Build history of the part. All positions in model axes, mm. Face numbers are marked on the shaded views. A direction names the side the tool comes from. Give positions to 0.01 mm unless a question says otherwise; leave off trailing zeros. Order: outer loops, then holes, each group sorted by start corner. A loop starts at its lowest first (then second) coordinate and runs counter-clockwise, first axis right, second up. Notation, with made-up numbers: (-17, 17) -> (23, 17) arc R20 cw to (23, 54) -> close; hole circle Ø6 at (-11.75, 15.25). An arc over 180 degrees is marked (long way). Write item = value, one per line. Start each with the question number.
from build123d import *

# Parameters (mm, degrees)
SKETCH1_W           = 140
SKETCH1_H           = 110
BOSS_EXTRUDE1_DEPTH = 5
SKETCH3_W           = 140
SKETCH3_H           = 110
SKETCH3_W_2         = 134
SKETCH3_H_2         = 104
BOSS_EXTRUDE2_DEPTH = 30
CUT_EXTRUDE3_DEPTH  = 5
FILLET1_R           = 3
SKETCH5_R           = 4
CUT_EXTRUDE4_DEPTH  = 2
SKETCH6_R           = 2
CUT_EXTRUDE5_DEPTH  = 5
FILLET2_R           = 10
CUT_EXTRUDE6_DEPTH  = 3
SKETCH9_W           = 32
SKETCH9_H           = 3
CUT_EXTRUDE7_DEPTH  = 3
SKETCH10_W          = 71
SKETCH10_H          = 23
CUT_EXTRUDE8_DEPTH  = 3


with BuildPart() as part:
    # Sketch1 → Boss-Extrude1 (new body)
    with BuildSketch(Plane(origin=(0, 0, 0), x_dir=(1, 0, 0), z_dir=(0, 1, 0))):
        with Locations((70, -55)):
            Rectangle(SKETCH1_W, SKETCH1_H)
    extrude(amount=BOSS_EXTRUDE1_DEPTH)

    # Sketch3 → Boss-Extrude2 (add)
    with BuildSketch(Plane(origin=(0, 5, 0), x_dir=(1, 0, 0), z_dir=(0, 1, 0))):
        with Locations((70, -55)):
            Rectangle(SKETCH3_W, SKETCH3_H)
        with Locations((70, -55)):
            Rectangle(SKETCH3_W_2, SKETCH3_H_2, mode=Mode.SUBTRACT)
    extrude(amount=BOSS_EXTRUDE2_DEPTH)

    # Sketch4 → Cut-Extrude3 (cut)
    with BuildSketch(Plane(origin=(0, 5, 0), x_dir=(1, 0, 0), z_dir=(0, 1, 0))):
        Polygon((23, -6), (23, -23), (6, -23), (6, -87), (23, -87), (23, -104), (117, -104), (117, -87), (134, -87), (134, -23), (117, -23), (117, -6), align=None)
    extrude(amount=-CUT_EXTRUDE3_DEPTH, mode=Mode.SUBTRACT)

    # Fillet1
    fillet1_edges = [part.edges().sort_by_distance(p)[0] for p in [
        (23, 2.5, 6),
        (117, 2.5, 6),
        (134, 2.5, 23),
        (134, 2.5, 87),
        (117, 2.5, 104),
        (23, 2.5, 104),
        (6, 2.5, 87),
        (6, 2.5, 23),
    ]]
    fillet(fillet1_edges, radius=FILLET1_R)

    # Sketch5 → Cut-Extrude4 (cut)
    with BuildSketch(Plane(origin=(0, 5, 0), x_dir=(1, 0, 0), z_dir=(0, 1, 0))):
        with Locations(Location((13, -13, 0), (0, 0, 270))):
            Circle(SKETCH5_R)
        with Locations(Location((13, -97, 0), (0, 0, 270))):
            Circle(SKETCH5_R)
    cut_extrude4 = extrude(amount=-CUT_EXTRUDE4_DEPTH, mode=Mode.SUBTRACT)

    # Sketch6 → Cut-Extrude5 (cut)
    with BuildSketch(Plane(origin=(0, 5, 0), x_dir=(1, 0, 0), z_dir=(0, 1, 0))):
        with Locations(Location((13, -13, 0), (0, 0, 270))):
            Circle(SKETCH6_R)
        with Locations(Location((13, -97, 0), (0, 0, 270))):
            Circle(SKETCH6_R)
    cut_extrude5 = extrude(amount=-CUT_EXTRUDE5_DEPTH, mode=Mode.SUBTRACT)

    # Mirror1: Cut-Extrude4, Cut-Extrude5 across plane
    add(cut_extrude4.mirror(Plane(origin=(70, 0, 0), x_dir=(0, 0, 1), z_dir=(1, 0, 0))), mode=Mode.SUBTRACT)
    add(cut_extrude5.mirror(Plane(origin=(70, 0, 0), x_dir=(0, 0, 1), z_dir=(1, 0, 0))), mode=Mode.SUBTRACT)

    # Fillet2
    fillet2_edges = [part.edges().sort_by_distance(p)[0] for p in [
        (117, 2.5, 23),
        (117, 2.5, 87),
        (23, 2.5, 87),
        (23, 2.5, 23),
    ]]
    fillet(fillet2_edges, radius=FILLET2_R)

    # Sketch8 → Cut-Extrude6 (cut)
    with BuildSketch(Plane(origin=(0, 0, 0), x_dir=(-1, 0, 0), z_dir=(0, 0, -1))):
        Polygon((-127, 31), (-127, 10), (-28, 10), (-28, 28), (-93, 28), (-93, 31), align=None)
    extrude(amount=-CUT_EXTRUDE6_DEPTH, mode=Mode.SUBTRACT)

    # Sketch9 → Cut-Extrude7 (cut)
    with BuildSketch(Plane(origin=(0, 0, 0), x_dir=(-1, 0, 0), z_dir=(0, 0, -1))):
        with Locations((-59, 33.5)):
            Rectangle(SKETCH9_W, SKETCH9_H)
    extrude(amount=-CUT_EXTRUDE7_DEPTH, mode=Mode.SUBTRACT)

    # Sketch10 → Cut-Extrude8 (cut)
    with BuildSketch(Plane.ZY):
        with Locations((55.5, 16.5)):
            Rectangle(SKETCH10_W, SKETCH10_H)
    extrude(amount=-CUT_EXTRUDE8_DEPTH, mode=Mode.SUBTRACT)


solid = part.part
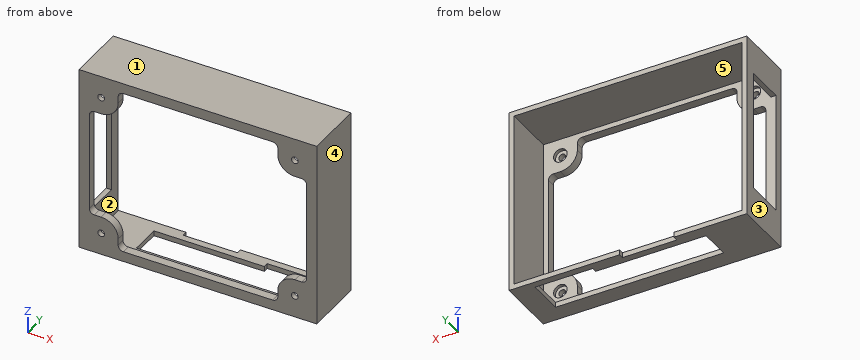
(1) Cut at A-A, the plane z = 35.5. Give the cut face in (x, y).
(2) Mould opens along Z. For the marked faces 1, 2 and 3 say: released by +Z, released by -Z, zero draft, split by the parting line, or undercut.
(3) 3-axis set-ups, long thin cutter, end or side, ignore diameter. For the marked faces 4 and 5: which of +Z, -Z, +X, -X, +Y, -Y reach the whole face in a straight line?
(4) Flat gauge pins, fed straight in: P1, Ø4, axis at y = 28.5, z = 87, coming from the -X side; P2, Ø9, axis at x = 127, z = 97, coming from the +Y side; P3, Ø3, axis at y = 17, z = 81.5, coming from the -X side; P4, Ø2.5, axis at x = 13, z = 97, coming from the -Y side. Where does each tip first touch, or does it go through?
(5) Cut at D-D, the plane x = 30. Give the cut face in (y, z).
(6) Wall check: line 1 (X direction, y = 3.75, z = 97); line 2 (X direction, y = 30, z = 68); line 3 (Z direction, x = 131.5, y = 7). Give the ranges that are in metal, low to high. Write a range as [from, to].
(7) Cut at C-C, the plane x = 49.5. Give the cut face in (y, z).
(8) Cut at B-B, the plane y = 18. Give the cut face in (x, z), plus the area to 3 significant figures.
Results:
q1.outline = (0, 0) -> (6, 0) -> (6, 5) -> (0, 5) -> close; (0, 28) -> (3, 28) -> (3, 35) -> (0, 35) -> close; (134, 0) -> (140, 0) -> (140, 35) -> (137, 35) -> (137, 5) -> (134, 5) -> close
q2.face_1 = released by +Z
q2.face_2 = undercut
q2.face_3 = zero draft
q3.face_4 = +Z, -Z, +X, +Y, -Y
q3.face_5 = +Y
q4.P1 = 0
q4.P2 = 5
q4.P3 = 137
q4.P4 = through
q5.outline = (0, 0) -> (10, 0) -> (10, 3) -> (5, 3) -> (5, 6) -> (0, 6) -> close; (0, 104) -> (5, 104) -> (5, 107) -> (35, 107) -> (35, 110) -> (0, 110) -> close; (28, 0) -> (35, 0) -> (35, 3) -> (28, 3) -> close
q6.line_1 = [0, 9], [17, 23], [117, 123], [131, 140]
q6.line_2 = [0, 3], [137, 140]
q6.line_3 = [0, 3], [107, 110]
q7.outline = (0, 0) -> (10, 0) -> (10, 3) -> (5, 3) -> (5, 6) -> (0, 6) -> close; (0, 104) -> (5, 104) -> (5, 107) -> (35, 107) -> (35, 110) -> (0, 110) -> close; (28, 0) -> (32, 0) -> (32, 3) -> (28, 3) -> close
q8.outline = (0, 0) -> (28, 0) -> (28, 3) -> (3, 3) -> (3, 20) -> (0, 20) -> close; (0, 91) -> (3, 91) -> (3, 107) -> (137, 107) -> (137, 3) -> (127, 3) -> (127, 0) -> (140, 0) -> (140, 110) -> (0, 110) -> close
q8.area = 954 mm2
